```python
from build123d import *

# Parameters (mm, degrees)
BOSS_EXTRUDE1_DEPTH                               = 3.5
FILLET1_R                                         = 5
FILLET2_R                                         = 1
CSK_FOR_M2_5_FLAT_HEAD_MACHINE_SCREW1_D           = 2.9
CSK_FOR_M2_5_FLAT_HEAD_MACHINE_SCREW1_CSINK_D     = 5.5
CSK_FOR_M2_5_FLAT_HEAD_MACHINE_SCREW1_CSINK_ANGLE = 90
SKETCH6_R                                         = 1.5
CUT_EXTRUDE3_DEPTH                                = 75.3320254
SKETCH7_W                                         = 23
SKETCH7_H                                         = 29
CUT_EXTRUDE4_DEPTH                                = 75.3320254
FILLET3_R                                         = 2.5
CUT_EXTRUDE2_DEPTH                                = 1


# Read off the part's stored shape, not the designer's step: Mirror1
with BuildPart() as part:
    # Sketch1 → Boss-Extrude1 (new body)
    with BuildSketch(Plane(origin=(0, 0, 0), x_dir=(1, 0, 0), z_dir=(0, 1, 0))):
        Polygon((0, 0), (23, 0), (30, -15), (52, -15), (52, 38), (47, 38), (40, 53), (0, 53), align=None)
    extrude(amount=BOSS_EXTRUDE1_DEPTH)

    # Fillet1
    fillet1_edges = [part.edges().sort_by_distance(p)[0] for p in [
        (40, 1.75, -53),
        (47, 1.75, -38),
        (30, 1.75, 15),
        (23, 1.75, 0),
    ]]
    fillet(fillet1_edges, radius=FILLET1_R)

    # Fillet2
    fillet2_edges = [part.edges().sort_by_distance(p)[0] for p in [
        (52, 1.75, -38),
        (52, 1.75, 15),
    ]]
    fillet(fillet2_edges, radius=FILLET2_R)

    # CSK for M2.5 Flat Head Machine Screw1 (through all)
    with Locations(Plane(origin=(0, 0, 0), x_dir=(-1, 0, 0), z_dir=(0, -1, 0))):
        with Locations((-5, 21), (-48, -3.5), (-48, 26.5)):
            CounterSinkHole(CSK_FOR_M2_5_FLAT_HEAD_MACHINE_SCREW1_D / 2, CSK_FOR_M2_5_FLAT_HEAD_MACHINE_SCREW1_CSINK_D / 2, counter_sink_angle=CSK_FOR_M2_5_FLAT_HEAD_MACHINE_SCREW1_CSINK_ANGLE)

    # Sketch6 → Cut-Extrude3 (cut, through all)
    with BuildSketch(Plane.XZ):
        with Locations(Location((48, 11.5, 0), (0, 0, 270))):
            Circle(SKETCH6_R)
        with Locations(Location((48, -34.5, 0), (0, 0, 270))):
            Circle(SKETCH6_R)
    extrude(amount=-CUT_EXTRUDE3_DEPTH, mode=Mode.SUBTRACT)

    # Sketch7 → Cut-Extrude4 (cut, through all)
    with BuildSketch(Plane(origin=(0, 3.5, 0), x_dir=(1, 0, 0), z_dir=(0, 1, 0))):
        with Locations((21.5, 24.5)):
            Rectangle(SKETCH7_W, SKETCH7_H)
    extrude(amount=-CUT_EXTRUDE4_DEPTH, mode=Mode.SUBTRACT)

    # Fillet3
    fillet3_edges = [part.edges().sort_by_distance(p)[0] for p in [
        (10, 1.75, -10),
        (10, 1.75, -39),
        (33, 1.75, -39),
        (33, 1.75, -10),
    ]]
    fillet(fillet3_edges, radius=FILLET3_R)

    # Mirror1: part across plane


with BuildPart() as part_1:
    add(part.part)
    add(part.part.mirror(Plane(origin=(0, 0, 0), x_dir=(0, 0, 1), z_dir=(1, 0, 0))))

    # Sketch2 → Cut-Extrude2 (cut)
    with BuildSketch(Plane(origin=(0, 3.5, 0), x_dir=(1, 0, 0), z_dir=(0, 1, 0))):
        with BuildLine():
            Line((-50.5, 36.5), (-50.5, -13.5))
            Line((-50.5, -13.5), (-33.184315119, -13.5))
            ThreePointArc((-33.184315119, -13.5), (-31.304201685, -12.952147265), (-30.012674129, -11.480099129))
            Line((-30.012674129, -11.480099129), (-25.705875291, -2.251244475))
            ThreePointArc((-25.705875291, -2.251244475), (-23.307324116, 0.482559207), (-19.815684881, 1.5))
            Line((-19.815684881, 1.5), (19.815684881, 1.5))
            ThreePointArc((19.815684881, 1.5), (23.307324116, 0.482559207), (25.705875291, -2.251244475))
            Line((25.705875291, -2.251244475), (30.012674129, -11.480099129))
            ThreePointArc((30.012674129, -11.480099129), (31.304201685, -12.952147265), (33.184315119, -13.5))
            Line((33.184315119, -13.5), (50.5, -13.5))
            Line((50.5, -13.5), (50.5, 36.5))
            Line((50.5, 36.5), (50.184315119, 36.5))
            ThreePointArc((50.184315119, 36.5), (46.692675884, 37.517440793), (44.294124709, 40.251244475))
            Line((44.294124709, 40.251244475), (39.987325871, 49.480099129))
            ThreePointArc((39.987325871, 49.480099129), (38.695798315, 50.952147265), (36.815684881, 51.5))
            Line((36.815684881, 51.5), (-36.815684881, 51.5))
            ThreePointArc((-36.815684881, 51.5), (-38.695798315, 50.952147265), (-39.987325871, 49.480099129))
            Line((-39.987325871, 49.480099129), (-44.294124709, 40.251244475))
            ThreePointArc((-44.294124709, 40.251244475), (-46.692675884, 37.517440793), (-50.184315119, 36.5))
            Line((-50.184315119, 36.5), (-50.5, 36.5))
        make_face()
    extrude(amount=-CUT_EXTRUDE2_DEPTH, mode=Mode.SUBTRACT)


solid = part_1.part
```
Could you check a few things on this model? Use its own coordinates, in mm. A direction names the side the tool comes from. Round coordinates to 2 decimals unless told otherwise and drop trailing zeros. Loops run counter-clockwise (first coordinate to the right, second up) from the corner with the lowest first, then second, coordinate; pieces in that order, holes last. Notation, with made-up numbers: M -13,-15 L 33,-15 A10 cw 33,3 Z; hole C 54,60.5 d11. An arc over 180 degrees is marked long. Put each result on its own line as item: value.
Q1. Imagine slicing it at A-A (x = 5). Write out the boundary of the cut face in (y, z), then the cut area to 3 significant figures.
Check result:
outline: M 0,-53 L 3.5,-53 L 3.5,-51.5 L 2.5,-51.5 L 2.5,-22.45 L 1.3,-22.45 L 0,-23.75 Z; M 0,-18.25 L 1.3,-19.55 L 2.5,-19.55 L 2.5,-1.5 L 3.5,-1.5 L 3.5,0 L 0,0 Z
area: 127 mm2
Q2. Imagine slicing it at D-D (z = 9). Write out the boundary of the cut face in (x, y), then the cut area to 3 significant figures.
Check result:
outline: M -52,0 L -27.2,0 L -27.2,3.5 L -28.86,3.5 L -28.86,2.5 L -50.5,2.5 L -50.5,3.5 L -52,3.5 Z; M 27.2,0 L 52,0 L 52,3.5 L 50.5,3.5 L 50.5,2.5 L 28.86,2.5 L 28.86,3.5 L 27.2,3.5 Z
area: 130 mm2
Q3. Imagine slicing it at B-B (z = -21). Write out the boundary of the cut face in (x, y).
Check result:
outline: M -52,0 L -33,0 L -33,2.5 L -50.5,2.5 L -50.5,3.5 L -52,3.5 Z; M -10,0 L -7.75,0 L -6.45,1.3 L -6.45,2.5 L -10,2.5 Z; M -3.55,1.3 L -2.25,0 L 2.25,0 L 3.55,1.3 L 3.55,2.5 L -3.55,2.5 Z; M 6.45,1.3 L 7.75,0 L 10,0 L 10,2.5 L 6.45,2.5 Z; M 33,0 L 52,0 L 52,3.5 L 50.5,3.5 L 50.5,2.5 L 33,2.5 Z
Q4. Thinking about a two-plate mould opening in Z: for faces 3 (the face through (-46.536, 1.232, 11.825)), 4 (the face through (26.47, 1.73, 7.44)), 5 (the face through (1, 0, -19)), which applies, released by +Z, released by -Z, zero draft, split by the parting line, or undercut?
Check result:
face 3: undercut
face 4: released by +Z
face 5: zero draft
Q5. Imagine slicing it at C-C (z = -32). Write out the boundary of the cut face in (x, y).
Check result:
outline: M -52,0 L -33,0 L -33,2.5 L -50.5,2.5 L -50.5,3.5 L -52,3.5 Z; M -10,0 L 10,0 L 10,2.5 L -10,2.5 Z; M 33,0 L 52,0 L 52,3.5 L 50.5,3.5 L 50.5,2.5 L 33,2.5 Z
Q6. For pin 1 (2.5 mm diameter, centred on x = -5, z = -21, fed in from +Y); pin 2 (2 mm diameter, centred on x = -17.5, y = 1.5, fed in from +Z); pin 3 (4 mm diameter, centred on x = -48, z = -34.5, fed in from +Y); pin 4 (4.5 mm diameter, centred on x = 48, z = -26.5, fed in from -Y), each with a flat end and sliding along its axis, tell me the tip position at first contact or that it passes through.
Check result:
pin 1: through
pin 2: z = 0
pin 3: y = 2.5
pin 4: y = 0.5
Q7. On a 3-axis mill with a long thin cutter (end or side, diameter ignored), from which of +Z, -Z, +X, -X, +Y, -Y can I reach the whole of each face in a straight line? I mean faces 1 (the face through (23.264, 3.007, -0.51)), 2 (the face through (-21, 1, -39)). Say none if no direction works.
Check result:
face 1: +Y
face 2: +Y, -Y
Q8. I need wall thicknesses on probe 1 along X at (y, z) = (0.65, -29.5); probe 2 along Z at (x, y) = (-5, 1.9); probe 3 along Z at (x, y) = (6.5, 3.15). Which ranges of each line are inside material? Lowest first, please.
Check result:
probe 1: -52 to -33, -10 to 10, 33 to 52
probe 2: -53 to -22.45, -19.55 to 0
probe 3: -53 to -51.5, -1.5 to 0
